For this review, take the finished solid that the model builds, in its own axes (mm). Round coordinates to 2 decimals unless told otherwise and drop trailing zeros. Order: outer loops, then holes, each group sorted by start corner. A loop starts at its lowest first (then second) coordinate and runs counter-clockwise, first axis right, second up. Notation, with made-up numbers: (58.25, -11) -> (82.25, -11) arc R21 cw to (82.25, 14) -> close; hole circle Ø6 at (45, -28.5). An arc over 180 degrees is marked (long way). Use a Markdown table: item, result. Add a question column.
1) Clearance check with flat-ended pins moving along their axes: P1, Ø6, axis at x = 143.5, y = 7, coming from the +Z side; P2, Ø2, axis at x = 92.5, z = 3, coming from the +Y side; P3, Ø5.5, axis at y = 0, z = 0, coming from the +X side. State where each tip first meets the part, or that it passes through.
2) Consider section A-A (x = 18.5). State the section outline as (y, z) points, plus the area to 3 significant figures.
3) Wall thickness on line 1 along Z through (x, y) = (-220.25, 0); line 2 along Y through (x, z) = (87, 0.25); line 3 along Z through (x, y) = (-81, 1): over which ranges is each line inside the solid? List them lowest first. Write a range as [from, to].
```python
from build123d import *


with BuildPart() as part:
    # Sketch1 → Revolve1 (revolve)
    with BuildSketch(Plane.XY, mode=Mode.PRIVATE) as revolve1_sk:
        Polygon((-235, 0), (235, 0), (235, 7.5), (227.5, 7.5), (227.5, 9), (-227.5, 9), (-227.5, 7.5), (-235, 7.5), align=None)
    revolve(revolve1_sk.sketch.rotate(Axis((-235, 0, 0), (1, 0, 0)), 180), axis=Axis((-235, 0, 0), (1, 0, 0)))

    # Sketch5 → M8 Tapped Hole2 (revolve, cut)
    with BuildSketch(Plane(origin=(235, 0, 0), x_dir=(0, 0, -1), z_dir=(0, 1, 0))):
        Polygon((0, 0), (0, 22.042926105), (3.4, 20), (3.4, 0.625), (4.025, 0), align=None)
    m8_tapped_hole2 = revolve(axis=Axis((241.35, 0, 0), (-1, 0, 0)), mode=Mode.SUBTRACT)

    # Mirror1: M8 Tapped Hole2 across plane
    add(m8_tapped_hole2.mirror(Plane(origin=(0, 0, 0), x_dir=(0, 0, 1), z_dir=(1, 0, 0))), mode=Mode.SUBTRACT)


solid = part.part
```
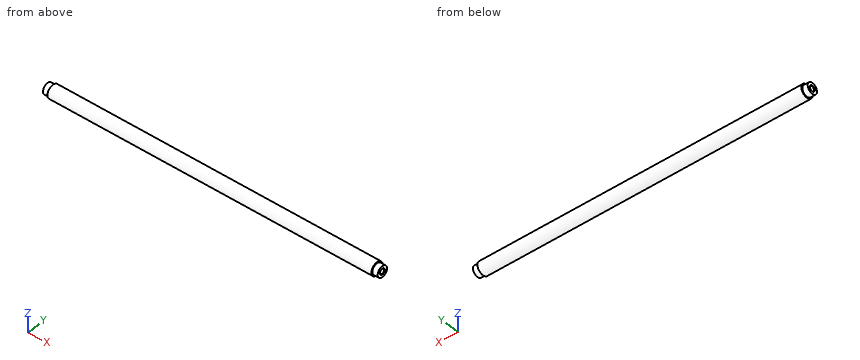
Results list:
| question | item | result |
|---|---|---|
| 1 | P1 | z = 8.06 |
| 1 | P2 | y = 8.77 |
| 1 | P3 | x = 214.61 |
| 2 | outline | circle Ø18 at (0, 0) |
| 2 | area | 254 mm2 |
| 3 | line 1 | [-9, -3.4], [3.4, 9] |
| 3 | line 2 | [-9, 9] |
| 3 | line 3 | [-8.94, 8.94] |
